from build123d import *

# Parameters (mm, degrees)
SKETCH1_R           = 3.175
BOSS_EXTRUDE1_DEPTH = 3.175
FILLET1_R           = 6.35


with BuildPart() as part:
    # Sketch1 → Boss-Extrude1 (new body)
    with BuildSketch(Plane.XY):
        Polygon((-353.401390066, 345.241574638), (-296.388854277, 341.280102322), (-302.110980955, 258.928661738), (-359.123516744, 262.890134053), align=None)
        with Locations((-306.771270757, 329.270895311)):
            Circle(SKETCH1_R, mode=Mode.SUBTRACT)
        with Locations((-341.61226485, 331.691795059)):
            Circle(SKETCH1_R, mode=Mode.SUBTRACT)
        with Locations((-345.573737165, 274.67925927)):
            Circle(SKETCH1_R, mode=Mode.SUBTRACT)
        with Locations((-310.732743072, 272.258359522)):
            Circle(SKETCH1_R, mode=Mode.SUBTRACT)
    extrude(amount=BOSS_EXTRUDE1_DEPTH)

    # Fillet1
    fillet1_edges = [part.edges().sort_by_distance(p)[0] for p in [
        (-353.401390066, 345.241574638, 1.5875),
        (-296.388854277, 341.280102322, 1.5875),
        (-302.110980955, 258.928661738, 1.5875),
        (-359.123516744, 262.890134053, 1.5875),
    ]]
    fillet(fillet1_edges, radius=FILLET1_R)


solid = part.part
Build history of the part. All positions in model axes, mm. Give positions to 0.01 mm unless a question says otherwise; leave off trailing zeros. Order: outer loops, then holes, each group sorted by start corner. A loop starts at its lowest first (then second) coordinate and runs counter-clockwise, first axis right, second up. Notation, with made-up numbers: M 48,45.25 L 102,45.25 A30 cw 102,72.25 Z; hole C 78,38 d6. An arc over 180 degrees is marked long. Put each result on its own line as item: value.
Item 1: Cut at D-D on x = -350.5. Write the cut outline in (y, z) (3 decimals), then the cut area to 3 significant figures.
Results are:
outline: M 262.291,0 L 344.067,0 L 344.067,3.175 L 262.291,3.175 Z
area: 260 mm2
Item 2: Cut at C-C on y = 309. Write the cut outline in (x, z) (3 decimals), then the cut area to 3 significant figures.
Results are:
outline: M -355.92,0 L -298.632,0 L -298.632,3.175 L -355.92,3.175 Z
area: 182 mm2
Item 3: Pull direction Y, two halves, no side cores. Call faces 1 (the face through (-342.545, 275.633, 1.565)), 2 (the face through (-327, 303, 3.175)), 3 (the face through (-330.31, 260.89, 1.57)): +Y half, -Y half, draft (parallel to the pull), parting line (faces both ways), or undercut.
Results are:
face 1: undercut
face 2: draft
face 3: -Y half
Item 4: Cut at A-A on x = -306.5. Write the cut outline in (y, z) (1 decimal), then the cut area to 3 significant figures.
Results are:
outline: M 259.5,0 L 326.1,0 L 326.1,3.2 L 259.5,3.2 Z; M 332.4,0 L 342,0 L 342,3.2 L 332.4,3.2 Z
area: 242 mm2
Item 5: Cut at B-B on z = 1.35. Write the cut outline in (x, y) (3 decimals).
Results are:
outline: M -358.683,269.225 A6.35 ccw -352.789,262.45 L -308.446,259.369 A6.35 ccw -301.671,265.263 L -296.829,334.945 A6.35 ccw -302.724,341.72 L -347.067,344.801 A6.35 ccw -353.842,338.907 Z; hole C -345.574,274.679 d6.35; hole C -341.612,331.692 d6.35; hole C -310.733,272.258 d6.35; hole C -306.771,329.271 d6.35
Item 6: Drop flat-ended pins along their axis: pin 1 Ø10 at (x, y) = (-339, 330) entering from +Z (3 decimals); pin 2 Ø1 at (y, z) = (288.5, 1) entering from -X; pin 3 Ø1.5 at (y, z) = (291.5, 2.5) entering from -X; pin 4 Ø1.5 at (y, z) = (306.5, 1.5) entering from -X. Give the stop position or say it passes through.
Results are:
pin 1: z = 3.175
pin 2: x = -357.38
pin 3: x = -357.19
pin 4: x = -356.15
Item 7: Wall check: probe 1 along Y at (x, z) = (-343.5, 0.95); probe 2 along Y at (x, z) = (-308.5, 1.15); probe 3 along X at (y, z) = (327.5, 0.1). Give the ranges that are in metal, low to high.
Results are:
probe 1: 261.8 to 272.28, 277.08 to 329.14, 334.24 to 344.55
probe 2: 259.37 to 270, 274.52 to 326.61, 331.93 to 342.12
probe 3: -354.63 to -309.41, -304.14 to -297.35
